```python
from build123d import *

# Parameters (mm, degrees)
SKETCH2_R           = 4
SKETCH2_W           = 52
SKETCH2_H           = 18
BOSS_EXTRUDE1_DEPTH = 6
FILLET1_R           = 5


with BuildPart() as part:
    # Sketch2 → Boss-Extrude1 (new body)
    with BuildSketch(Plane(origin=(0, 0, 0), x_dir=(0, 0, -1), z_dir=(1, 0, 0))):
        with BuildLine():
            Line((-10, 0), (-10, 180))
            ThreePointArc((-10, 180), (0, 190), (10, 180))
            Line((10, 180), (10, 0))
            ThreePointArc((10, 0), (0, -10), (-10, 0))
        make_face()
        Circle(SKETCH2_R, mode=Mode.SUBTRACT)
        with Locations((0, 180)):
            Circle(SKETCH2_R, mode=Mode.SUBTRACT)
        with Locations((0, 40)):
            Rectangle(SKETCH2_W, SKETCH2_H)
        with Locations((-16, 40)):
            Circle(SKETCH2_R, mode=Mode.SUBTRACT)
        with Locations((16, 40)):
            Circle(SKETCH2_R, mode=Mode.SUBTRACT)
    extrude(amount=BOSS_EXTRUDE1_DEPTH)

    # Fillet1
    fillet1_edges = [part.edges().sort_by_distance(p)[0] for p in [
        (3, 49, 10),
        (3, 49, -10),
        (3, 49, -26),
        (3, 31, -26),
        (3, 31, -10),
        (3, 31, 10),
        (3, 31, 26),
        (3, 49, 26),
    ]]
    fillet(fillet1_edges, radius=FILLET1_R)


solid = part.part
```
Source: CAD feature listing. Evaluate the final solid. Frame: model axes, mm. A direction names the side the tool comes from. Give positions to 0.01 mm unless a question says otherwise; leave off trailing zeros. Order: outer loops, then holes, each group sorted by start corner. A loop starts at its lowest first (then second) coordinate and runs counter-clockwise, first axis right, second up.
(1) Material intervals for line 1 along Y through (x, z) = (4.35, 0); line 2 along Z through (x, y) = (1.2, 179.5); line 3 along Y through (x, z) = (3.1, -16), sorted ascending.
(2) Section query A-A (z = 0). Return the cut outline in (x, y).
(3) Access query for faces 4 (the face through (3, 49, -18)), 5 (the face through (3, 116, 10)), 6 (the face through (3, 31, 18)). Directions: +Z, -Z, +X, -X, +Y, -Y. A direction counts if a zero-diameter tool reaches every point of the face in a straight line with its end or side. Return the directions, or none.
(4) Section query B-B (y = 40). Return the cut outline in (x, z), plus the area to 3 significant figures.
(5) Contact query for flat-ended pins moving along their axis: P1, Ø1.5, axis at x = 2, z = 20, coming from the -Y side; P2, Ø2, axis at x = 4, y = 157, coming from the -Z side; P3, Ø6.5, axis at y = 40, z = 16, coming from the -X side; P4, Ø1.8, axis at x = 2.5, z = 19.5, coming from the +Y side. Output: stop coordinate, or through.
(6) Pull-direction query (Z, two-part tool) for faces 1 (the face through (3, 50, -12)), 2 (the face through (6, 91, 0)), 3 (the face through (2.958, -3.905, 0.867)); classes: +Z half, -Z half, draft (parallel to the pull), parting line (faces both ways), or undercut.
(7) Section query C-C (x = 1.5). Return the cut outline in (y, z), plus the area to 3 significant figures.
Outcome:
1. line 1: y = -10 to -4, 4 to 176, 184 to 190
1. line 2: z = -10 to -3.97, 3.97 to 10
1. line 3: y = 31 to 36, 44 to 49
2. outline: (0, -10) - (6, -10) - (6, -4) - (0, -4) - close; (0, 4) - (6, 4) - (6, 176) - (0, 176) - close; (0, 184) - (6, 184) - (6, 190) - (0, 190) - close
3. face 4: -Z, +X, -X, +Y
3. face 5: +Z, +X, -X, +Y
3. face 6: +Z, +X, -X, -Y
4. outline: (0, -26) - (6, -26) - (6, -20) - (0, -20) - close; (0, -12) - (6, -12) - (6, 12) - (0, 12) - close; (0, 20) - (6, 20) - (6, 26) - (0, 26) - close
4. area: 216 mm2
5. P1: stops at y = 31
5. P2: stops at z = -10
5. P3: passes through
5. P4: stops at y = 49
6. face 1: -Z half
6. face 2: draft
6. face 3: undercut
7. outline: (0, -10) - (26, -10) arc R5 cw to (31, -15) - (31, -21) arc R5 ccw to (36, -26) - (44, -26) arc R5 ccw to (49, -21) - (49, -15) arc R5 cw to (54, -10) - (180, -10) arc R10 ccw to (180, 10) - (54, 10) arc R5 cw to (49, 15) - (49, 21) arc R5 ccw to (44, 26) - (36, 26) arc R5 ccw to (31, 21) - (31, 15) arc R5 cw to (26, 10) - (0, 10) arc R10 ccw to start; hole circle Ø8 at (0, 0); hole circle Ø8 at (40, -16); hole circle Ø8 at (40, 16); hole circle Ø8 at (180, 0)
7. area: 4,290 mm2
